```python
from build123d import *

# Parameters (mm, degrees)
SKETCH3_R           = 6.75
CUT_EXTRUDE1_DEPTH  = 15
SKETCH4_W           = 5.8
SKETCH4_H           = 5.8
BOSS_EXTRUDE1_DEPTH = 15
SKETCH6_R           = 7
BOSS_EXTRUDE2_DEPTH = 23
SKETCH7_R           = 3.5
CUT_EXTRUDE2_DEPTH  = 15
CUT_EXTRUDE3_DEPTH  = 15


with BuildPart() as part:
    # Sketch2 → Revolve2 (revolve)
    with BuildSketch(Plane.XY):
        Polygon((19.5, 0), (19.5, 7), (8, 7), (8, 27), (0, 27), (0, 0), align=None)
    revolve(axis=Axis((0, 96.27972973, 0), (0, -1, 0)))

    # Sketch3 → Cut-Extrude1 (cut)
    with BuildSketch(Plane(origin=(0, 27, 0), x_dir=(1, 0, 0), z_dir=(0, 1, 0))):
        Circle(SKETCH3_R)
    extrude(amount=-CUT_EXTRUDE1_DEPTH, mode=Mode.SUBTRACT)

    # Sketch4 → Boss-Extrude1 (add)
    with BuildSketch(Plane(origin=(0, 12, 0), x_dir=(1, 0, 0), z_dir=(0, 1, 0))):
        with Locations((0.004761868, -0.002625461)):
            Rectangle(SKETCH4_W, SKETCH4_H)
    extrude(amount=BOSS_EXTRUDE1_DEPTH)

    # Sketch6 → Boss-Extrude2 (add)
    with BuildSketch(Plane.XZ):
        Circle(SKETCH6_R)
    extrude(amount=BOSS_EXTRUDE2_DEPTH)

    # Sketch7 → Cut-Extrude2 (cut)
    with BuildSketch(Plane.XZ.offset(23)):
        Circle(SKETCH7_R)
    extrude(amount=-CUT_EXTRUDE2_DEPTH, mode=Mode.SUBTRACT)

    # Sketch8 → Cut-Extrude3 (cut)
    with BuildSketch(Plane.XZ.offset(23)):
        Polygon((-5.3, 1.5), (-1.5, 1.5), (-1.5, 5.3), (1.5, 5.3), (1.5, 1.5), (5.3, 1.5), (5.3, -1.5), (1.5, -1.5), (1.5, -5.3), (-1.5, -5.3), (-1.5, -1.5), (-5.3, -1.5), align=None)
    extrude(amount=-CUT_EXTRUDE3_DEPTH, mode=Mode.SUBTRACT)


solid = part.part
```
Work out the finished part from the listing and answer in its coordinate system (mm). A direction names the side the tool comes from. Round coordinates to 2 decimals unless told otherwise and drop trailing zeros. Write each loop counter-clockwise with the first axis right and the second up, starting at its lowest first coordinate (ties: lowest second). Pieces come first, ordered by that corner, then holes.
1) Determine the mould class of faces 1 (the face through (-1.73, 17.14, -7.81)), 2 (the face through (0, 19, -2.897)), 3 (the face through (-4, 27, -6)) for opening direction Z: pulls with the +Z half, pulls with the -Z half, needs draft (parallel to the pull), parting line crosses it, or undercut.
2) A cutting plane is placed at C-C on z = 0. Determine the outline of the cut face in (x, y), and give its area (4 significant figures).
3) Which of the six approach directions +Z, -Z, +X, -X, +Y, -Y give full straight-line access (tool end or side, diameter ignored) to faces 4 (the face through (-2.49, -15.6, -2.46)), 5 (the face through (-2.895, 19, 0))?
4) Flat-ended cylindrical pins translate along their axes: P1, Ø0.6, axis at y = -16, z = -4, coming from the +X side; P2, Ø1.7, axis at x = 3.5, y = -14, coming from the -Z side; P3, Ø2.5, axis at x = -4.5, y = -12, coming from the -Z side. Find the tip coordinate at first contact, or state that the pin passes through.
5) A cutting plane is placed at A-A on y = 17. Determine the outline of the cut face in (x, z).
6) A cutting plane is placed at D-D on x = 0. Determine the outline of the cut face in (y, z), and give its area (4 significant figures).
7) Consider probe 1 along Z at (x, y) = (0, 17); probe 2 along Y at (x, z) = (-12, 14); probe 3 along Z at (x, y) = (-3, 16). Determine where each line is inside the solid, lowest interval first.
8) A cutting plane is placed at B-B on y = -15. Determine the outline of the cut face in (x, z).
Entries:
1. face 1: parting line crosses it
1. face 2: undercut
1. face 3: needs draft
2. outline: (-19.5, 0) - (-7, 0) - (-7, -23) - (-5.3, -23) - (-5.3, -8) - (5.3, -8) - (5.3, -23) - (7, -23) - (7, 0) - (19.5, 0) - (19.5, 7) - (8, 7) - (8, 27) - (6.75, 27) - (6.75, 12) - (2.9, 12) - (2.9, 27) - (-2.9, 27) - (-2.9, 12) - (-6.75, 12) - (-6.75, 27) - (-8, 27) - (-8, 7) - (-19.5, 7) - close
2. area: 640.5 mm2
3. face 4: -Y
3. face 5: +Y
4. P1: stops at x = 5.94
4. P2: stops at z = -6.48
4. P3: stops at z = -6.2
5. outline: circle Ø16 at (0, 0); (-2.9, -2.9) - (2.9, -2.9) - (2.9, 2.9) - (-2.9, 2.9) - close; hole circle Ø13.5 at (0, 0)
6. outline: (-23, -7) - (0, -7) - (0, -19.5) - (7, -19.5) - (7, -8) - (27, -8) - (27, -6.75) - (12, -6.75) - (12, -2.9) - (27, -2.9) - (27, 2.9) - (12, 2.9) - (12, 6.75) - (27, 6.75) - (27, 8) - (7, 8) - (7, 19.5) - (0, 19.5) - (0, 7) - (-23, 7) - (-23, 5.3) - (-8, 5.3) - (-8, -5.3) - (-23, -5.3) - close
6. area: 640.5 mm2
7. probe 1: z = -8 to -6.75, -2.9 to 2.9, 6.75 to 8
7. probe 2: y = 0 to 7
7. probe 3: z = -7.42 to -6.05, 6.05 to 7.42
8. outline: circle Ø14 at (0, 0); hole (-5.3, -1.5) - (-3.16, -1.5) arc R3.5 ccw to (-1.5, -3.16) - (-1.5, -5.3) - (1.5, -5.3) - (1.5, -3.16) arc R3.5 ccw to (3.16, -1.5) - (5.3, -1.5) - (5.3, 1.5) - (3.16, 1.5) arc R3.5 ccw to (1.5, 3.16) - (1.5, 5.3) - (-1.5, 5.3) - (-1.5, 3.16) arc R3.5 ccw to (-3.16, 1.5) - (-5.3, 1.5) - close
